Model file for the job. Use its own axes, mm. Coordinates: 2 decimals unless noted, no trailing zeros. Write each loop counter-clockwise with the first axis right and the second up, starting at its lowest first coordinate (ties: lowest second). Pieces come first, ordered by that corner, then holes. Notation, with made-up numbers: M 50,-23.75 L 73,-23.75 A18 ccw 73,-16.75 Z; hole C 61,-5.75 d7. An arc over 180 degrees is marked long. One line per question, with ' | ' between items. Start each with the question number.
(1) Wall check: probe 1 along Y at (x, z) = (-29.5, 0.45) (3 decimals); probe 2 along Y at (x, z) = (-11.5, 2.7) (3 decimals); probe 3 along X at (y, z) = (4, 4.9) (3 decimals). Give the ranges that are in metal, low to high.
(2) Cut at A-A (x = -8). Write the cut outline in (y, z) (3 decimals).
(3) Flat gauge pins, fed straight in: pin 1 Ø1 at (x, z) = (-16.5, 2.5) entering from -Y (3 decimals); pin 2 Ø1.7 at (y, z) = (4.5, 4) entering from -X (3 decimals); pin 3 Ø3.5 at (x, y) = (30.625, 17.125) entering from +Z. Where does each tip first touch, or does it go through?
(4) Cut at B-B (y = -7). Write the cut outline in (x, z) (3 decimals).
(5) Cut at D-D (x = -28). Write the cut outline in (y, z) (3 decimals), plus the area to 3 significant figures.
(6) Cut at C-C (z = 2.4). Write the cut outline in (x, y) (3 decimals).
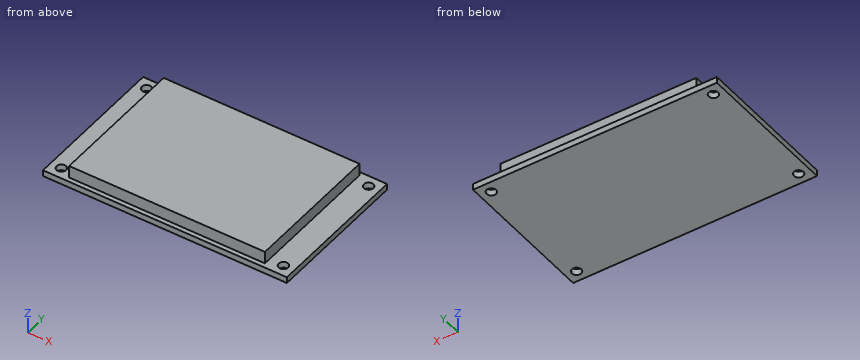
from build123d import *

# Parameters (mm, degrees)
SKETCH_1_W        = 67.25
SKETCH_1_H        = 40.25
EXTRUDE_1_DEPTH   = 1.7
SKETCH_2_W        = 54
SKETCH_2_H        = 38
EXTRUDE_2_DEPTH   = 3.4
HOLE_WIZARD_M21_D = 2.6


with BuildPart() as part:
    # Эскиз1 → Бобышка-Вытянуть1 (new body)
    with BuildSketch(Plane.XY):
        Rectangle(SKETCH_1_W, SKETCH_1_H)
    extrude(amount=EXTRUDE_1_DEPTH)

    # Эскиз2 → Бобышка-Вытянуть2 (add)
    with BuildSketch(Plane.XY.offset(1.7)):
        with Locations((-0.275, 0.125)):
            Rectangle(SKETCH_2_W, SKETCH_2_H)
    extrude(amount=EXTRUDE_2_DEPTH)

    # Отверстие с зазором M21 (through all)
    with Locations(Plane.XY.offset(1.7)):
        with Locations((-30.625, 17.125), (-30.625, -17.125), (30.625, -17.125), (30.625, 17.125)):
            Hole(HOLE_WIZARD_M21_D / 2)


solid = part.part
Filled in:
1) probe 1: -20.125 to -17.776, -16.474 to 16.474, 17.776 to 20.125 | probe 2: -18.875 to 19.125 | probe 3: -27.275 to 26.725
2) outline: M -20.125,0 L 20.125,0 L 20.125,1.7 L 19.125,1.7 L 19.125,5.1 L -18.875,5.1 L -18.875,1.7 L -20.125,1.7 Z
3) pin 1: y = -18.875 | pin 2: x = -27.275 | pin 3: z = 1.7
4) outline: M -33.625,0 L 33.625,0 L 33.625,1.7 L 26.725,1.7 L 26.725,5.1 L -27.275,5.1 L -27.275,1.7 L -33.625,1.7 Z
5) outline: M -20.125,0 L 20.125,0 L 20.125,1.7 L -20.125,1.7 Z | area: 68.4 mm²
6) outline: M -27.275,-18.875 L 26.725,-18.875 L 26.725,19.125 L -27.275,19.125 Z
